The drawing under review shows one solid part. Ordinate dimensions are in mm from its lowest x, y, z. A direction names the side the tool comes from. Round coordinates to 2 decimals unless told otherwise and drop trailing zeros. Order: outer loops, then holes, each group sorted by start corner. A loop starts at its lowest first (then second) coordinate and runs counter-clockwise, first axis right, second up. Notation, with made-up numbers: (74, 42.5) -> (107, 42.5) arc R12 ccw to (107, 65.5) -> close; hole circle Ø10 at (25, -38). An arc over 180 degrees is marked (long way). Use a Markdown table: item, result. Add a question column.
1) Wall thickness on line 1 along X through (y, z) = (38.5, 21); line 2 along Y through (x, z) = (61, 19.5); line 3 along Z through (x, y) = (30.6, 1.6): over which ranges is each line inside the solid? List them lowest first. Write a range as [from, to].
2) Consider section B-B (x = 26). State the section outline as (y, z) points, plus the area to 3 significant figures.
3) Consider section D-D (z = 15.25). State the section outline as (x, y) points.
4) Consider section C-C (y = 25). State the section outline as (x, z) points, plus the area to 3 significant figures.
5) Clearance check with flat-ended pins moving along their axes: P1, Ø8, axis at x = 61, y = 46.5, coming from the +Z side; P2, Ø8, axis at x = 20.9, z = 10.4, coming from the +Y side. State where each tip first meets the part, or that it passes through.
6) Machinability: for the marked faces 1 and 2, which of the approach directions +Z, -Z, +X, -X, +Y, -Y give a long, thin tool a straight path to every point of the face, cutting with its end or side? Answer none if there is none.
7) Consider section A-A (x = 11.2). State the section outline as (y, z) points.
8) Draft analysis for pull direction X (two halves, no side actions). For the marked faces 3, 4, 5 and 6, state which applies: pulls with the +X half, pulls with the -X half, needs draft (parallel to the pull), parting line crosses it, or undercut.
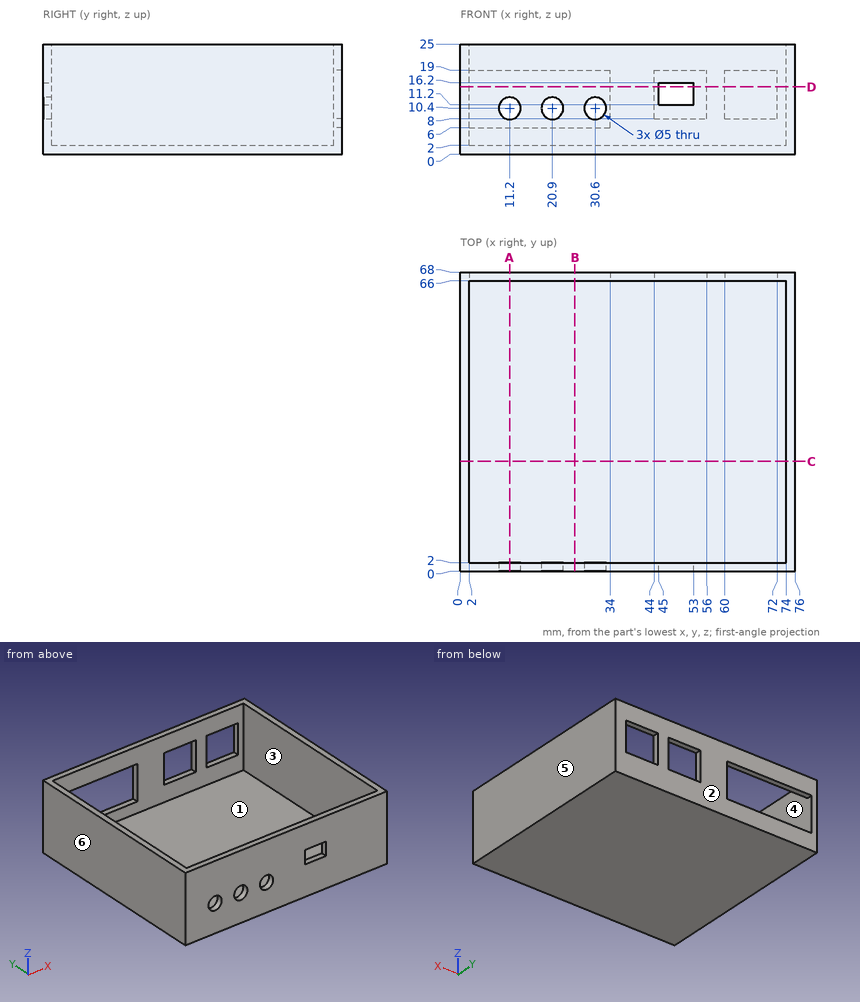
Results list:
| question | item | result |
|---|---|---|
| 1 | line 1 | [0, 2], [74, 76] |
| 1 | line 2 | [0, 2], [66, 68] |
| 1 | line 3 | [0, 7.9], [12.9, 25] |
| 2 | outline | (0, 0) -> (68, 0) -> (68, 6) -> (66, 6) -> (66, 2) -> (2, 2) -> (2, 25) -> (0, 25) -> close; (66, 19) -> (68, 19) -> (68, 25) -> (66, 25) -> close |
| 2 | area | 202 mm2 |
| 3 | outline | (0, 0) -> (45, 0) -> (45, 2) -> (2, 2) -> (2, 68) -> (0, 68) -> close; (34, 66) -> (44, 66) -> (44, 68) -> (34, 68) -> close; (53, 0) -> (76, 0) -> (76, 68) -> (72, 68) -> (72, 66) -> (74, 66) -> (74, 2) -> (53, 2) -> close; (56, 66) -> (60, 66) -> (60, 68) -> (56, 68) -> close |
| 4 | outline | (0, 0) -> (76, 0) -> (76, 25) -> (74, 25) -> (74, 2) -> (2, 2) -> (2, 25) -> (0, 25) -> close |
| 4 | area | 244 mm2 |
| 5 | P1 | z = 2 |
| 5 | P2 | y = 2 |
| 6 | face 1 | +Z |
| 6 | face 2 | +Z, -Z, +X, -X, +Y |
| 7 | outline | (0, 0) -> (68, 0) -> (68, 6) -> (66, 6) -> (66, 2) -> (2, 2) -> (2, 7.9) -> (0, 7.9) -> close; (0, 12.9) -> (2, 12.9) -> (2, 25) -> (0, 25) -> close; (66, 19) -> (68, 19) -> (68, 25) -> (66, 25) -> close |
| 8 | face 3 | undercut |
| 8 | face 4 | undercut |
| 8 | face 5 | pulls with the +X half |
| 8 | face 6 | pulls with the -X half |
